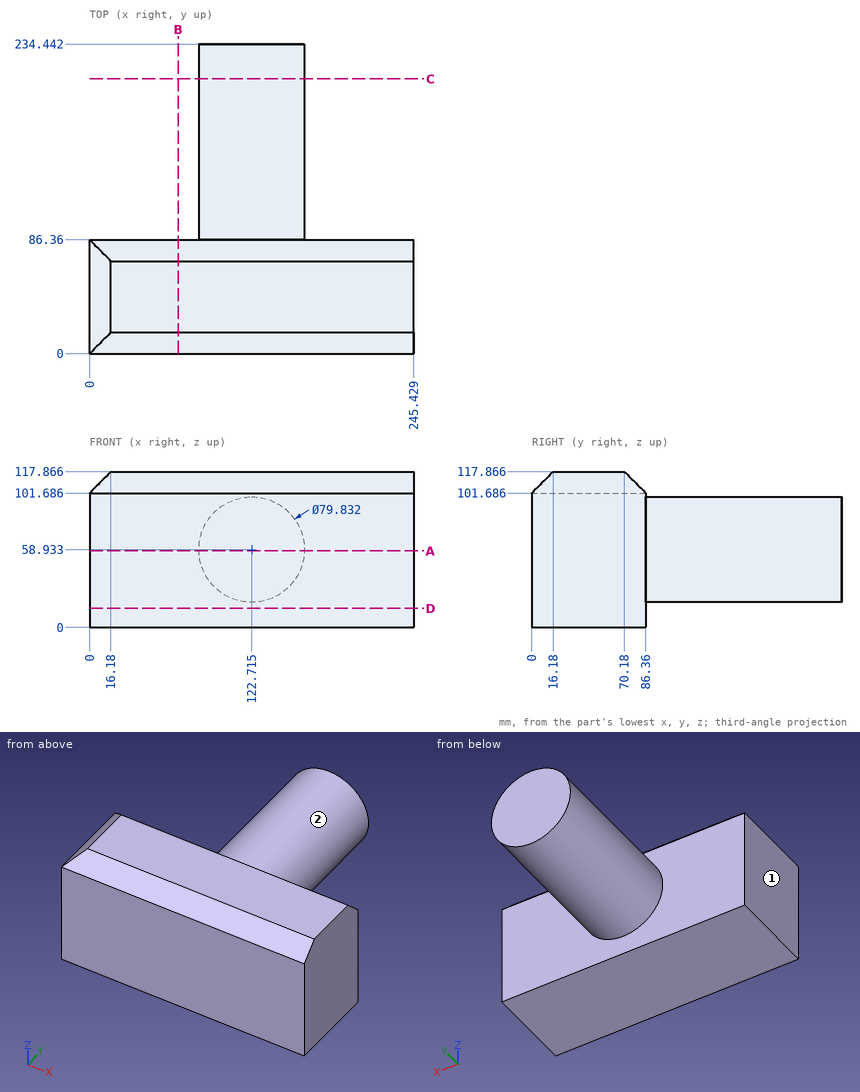
Drawing for the job (mm, zero at the part's lowest x, y, z). A direction names the side the tool comes from. Round coordinates to 2 decimals unless told otherwise and drop trailing zeros. Write each loop counter-clockwise with the first axis right and the second up, starting at its lowest first coordinate (ties: lowest second). Pieces come first, ordered by that corner, then holes. Notation, with made-up numbers: M 63.25,8 L 78.25,8 A28 cw 78.25,31 Z; hole C -2.5,31 d9. An arc over 180 degrees is marked long. Answer as a JSON object with one key per item and string values. Group by question number.
(1) Flat gauge pin, fed straight in: pin 1 (2 mm diameter, centred on y = 106, z = 25.5, fed in from -X) (1 decimal). Where does the tip first touch, or does it go through?
(2) Cut at A-A (z = 58). Give the cut face in (x, y).
(3) Drill centre lines: L1, parallel to Y at x = 85.5, z = 88; L2, parallel to X at y = 222, z = 50.5; L3, parallel to Z at x = 145, y = 85 (1 decimal). Where is each one in solid material? Low to high.
(4) Cut at D-D (z = 14.5). Give the cut face in (x, y), and give its area (3 significant figures).
(5) Cut at C-C (y = 208). Give the cut face in (x, z) (1 decimal).
(6) Cut at B-B (x = 67). Give the cut face in (y, z) (1 decimal).
(7) Which spindle directions (+Z, -Z, +X, -X, +Y, -Y) get a long thin tool onto all of the face, cutting with end or side? Do the marked faces 1 and 2. Say none if no direction does.
Responses:
{
 "1": {"pin 1": "stops at x = 99.4"},
 "2": {"outline": "M 0,0 L 245.43,0 L 245.43,86.36 L 162.62,86.36 L 162.62,234.44 L 82.81,234.44 L 82.81,86.36 L 0,86.36 Z"},
 "3": {"L1": "y = 0 to 86.36", "L2": "x = 83.7 to 161.73", "L3": "z = 0 to 103"},
 "4": {"outline": "M 0,0 L 245.43,0 L 245.43,86.36 L 0,86.36 Z", "area": "21,200 mm2"},
 "5": {"outline": "C 122.7,58.9 d79.8"},
 "6": {"outline": "M 0,0 L 86.4,0 L 86.4,101.7 L 70.2,117.9 L 16.2,117.9 L 0,101.7 Z"},
 "7": {"face 1": "+Z, -Z, -X, +Y, -Y", "face 2": "+Y"}
}
